Could you check a few things on this model? Use its own coordinates, in mm. A direction names the side the tool comes from. Round coordinates to 2 decimals unless told otherwise and drop trailing zeros. Loops run counter-clockwise (first coordinate to the right, second up) from the corner with the lowest first, then second, coordinate; pieces in that order, holes last. Notation, with made-up numbers: (24, 66) -> (45, 66) arc R18 cw to (45, 87) -> close; hole circle Ø5 at (66.5, 55). An arc over 180 degrees is marked (long way). One line per item, written item: value.
```python
from build123d import *

# Parameters (mm, degrees)
F0_R     = 40.044242968
F0_R_2   = 3.8023358025
F1_DEPTH = 6.35
F2_R     = 25.1375995998
F3_DEPTH = 50.8
F5_R     = 24.3470793068
F6_DEPTH = 114.301


with BuildPart() as f1:
    # F0 (on Top) → F1 (new body)
    with BuildSketch(Plane.XY):
        Circle(F0_R)
        with Locations((-27.5898085333, -15.9289833836)):
            Circle(F0_R_2, mode=Mode.SUBTRACT)
        with Locations((0, -31.8579667672)):
            Circle(F0_R_2, mode=Mode.SUBTRACT)
        with Locations((27.5898085333, -15.9289833836)):
            Circle(F0_R_2, mode=Mode.SUBTRACT)
        with Locations((-27.5898085333, 15.9289833836)):
            Circle(F0_R_2, mode=Mode.SUBTRACT)
        with Locations((27.5898085333, 15.9289833836)):
            Circle(F0_R_2, mode=Mode.SUBTRACT)
        with Locations((0, 31.8579667672)):
            Circle(F0_R_2, mode=Mode.SUBTRACT)
    extrude(amount=F1_DEPTH)

    # F2 (on face) → F3 (join)
    with BuildSketch(Plane.XY.offset(6.35)):
        Circle(F2_R)
    extrude(amount=F3_DEPTH)

    # F4: F1 across face


with BuildPart() as f1_1:
    add(f1.part)
    add(f1.part.mirror(Plane.XY.offset(57.15)))

    # F5 (on face) → F6 (cut, through all)
    with BuildSketch(Plane(origin=(0, 0, 0), x_dir=(1, 0, 0), z_dir=(0, 0, -1))):
        Circle(F5_R)
    extrude(amount=-F6_DEPTH, mode=Mode.SUBTRACT)


solid = f1_1.part
```
(1) Imagine slicing it at B-B on x = 0. Give the number of separate pieces and of enclosed holes in the cut face, then the cut area to 3 significant figures.
Results below:
separate pieces: 6
enclosed holes: 0
area: 366 mm²
(2) For pin 1 Ø5 at (y, z) = (24.5, 97) entering from -X; pin 2 Ø3 at (y, z) = (-19, 22.5) entering from +X; pin 3 Ø12 at (y, z) = (-3.5, 90) entering from +X, each with a flat end and sliding along its axis, tell me the tip position at first contact or that it passes through.
Results below:
pin 1: stops at x = -12.16
pin 2: stops at x = 18.05
pin 3: stops at x = 25.14
(3) Imagine slicing it at D-D on z = 77. Write out the boundary of the cut face in (x, y).
Results below:
outline: circle Ø50.28 at (0, 0); hole circle Ø48.69 at (0, 0)
(4) Imagine slicing it at A-A on y = 0. Write out the boundary of the cut face in (x, z), then the cut area to 3 significant figures.
Results below:
outline: (-40.04, 0) -> (-24.35, 0) -> (-24.35, 114.3) -> (-40.04, 114.3) -> (-40.04, 107.95) -> (-25.14, 107.95) -> (-25.14, 6.35) -> (-40.04, 6.35) -> close; (24.35, 0) -> (40.04, 0) -> (40.04, 6.35) -> (25.14, 6.35) -> (25.14, 107.95) -> (40.04, 107.95) -> (40.04, 114.3) -> (24.35, 114.3) -> close
area: 559 mm²
(5) Imagine slicing it at C-C on x = 13. Write out the boundary of the cut face in (y, z), then the cut area to 3 significant figures.
Results below:
outline: (-37.88, 0) -> (-20.59, 0) -> (-20.59, 114.3) -> (-37.88, 114.3) -> (-37.88, 107.95) -> (-21.52, 107.95) -> (-21.52, 6.35) -> (-37.88, 6.35) -> close; (20.59, 0) -> (37.88, 0) -> (37.88, 6.35) -> (21.52, 6.35) -> (21.52, 107.95) -> (37.88, 107.95) -> (37.88, 114.3) -> (20.59, 114.3) -> close
area: 628 mm²
(6) We'd pull the mould along Z, two halves only. Please class faces 3 (the face through (17, 18, 0)), 4 (the face through (26.77, -19.64, 3.13)), 5 (the face through (26, 1, 6.35)): +Z half, -Z half, draft (parallel to the pull), parting line (faces both ways), or undercut.
Results below:
face 3: -Z half
face 4: draft
face 5: undercut
(7) Please list where these lines run through material, in increasing order: L1, parallel to Y at x = 0, z = 3.75; L2, parallel to X at y = 1, z = 44.5; L3, parallel to Z at x = 33, y = -20.
Results below:
L1: y = -40.04 to -35.66, -28.06 to -24.35, 24.35 to 28.06, 35.66 to 40.04
L2: x = -25.12 to -24.33, 24.33 to 25.12
L3: z = 0 to 6.35, 107.95 to 114.3
(8) On a 3-axis mill with a long thin cutter (end or side, diameter ignored), from which of +Z, -Z, +X, -X, +Y, -Y can I reach the whole of each face in a straight line? I mean faces 1 (the face through (26, 1, 107.95)), 2 (the face through (-31.39, 16.1, 111.17)). Say none if no direction works.
Results below:
face 1: none
face 2: +Z, -Z
